```python
from build123d import *

# Parameters (mm, degrees)
F0_W     = 20
F0_H     = 20
F1_DEPTH = 20
F3_D     = 2
F5_D     = 2
F7_D     = 2


with BuildPart() as f1:
    # F0 (on Front) → F1 (new body)
    with BuildSketch(Plane.XZ):
        with Locations((10, 10)):
            Rectangle(F0_W, F0_H)
    extrude(amount=F1_DEPTH)

    # F3 (through all)
    with Locations(Plane.XZ.offset(20)):
        with Locations((10, 10)):
            Hole(F3_D / 2)

    # F5 (through all)
    with Locations(Plane.XY.offset(20)):
        with Locations((4.899733, -4.899733), (10, -10), (15.100267, -15.100267)):
            Hole(F5_D / 2)

    # F7 (through all)
    with Locations(Plane.YZ.offset(20)):
        with Locations((-10, 10), (-15.680383, 15.680383), (-15.680383, 4.319617), (-4.319617, 4.319617), (-4.319617, 15.680383)):
            Hole(F7_D / 2)


solid = f1.part
```
Geometry check sheet. Reference: the model listing, model coordinates, mm. Round coordinates to 2 decimals unless told otherwise and drop trailing zeros. Loops run counter-clockwise (first coordinate to the right, second up) from the corner with the lowest first, then second, coordinate; pieces in that order, holes last. Notation, with made-up numbers: M -29.5,-22.75 L 11.5,-22.75 A5 cw 11.5,-13.75 Z; hole C 56,-0.75 d1. An arc over 180 degrees is marked long. Return JSON: item names as keys, results as strings. Group by question number.
(1) Section check A-A, the plane y = -10. Enter the section's corners in (x, z).
(2) Section check C-C, the plane z = 15.25. Enter the section's corners in (x, y), and give its area (3 significant figures).
(3) Section check B-B, the plane x = 14.5. Enter the section's corners in (y, z), and give its area (3 significant figures).
(4) Scan lines: line 1 along Y through (x, z) = (3, 4.25); line 2 along Z through (x, y) = (10, -6); line 3 along Y through (x, z) = (3.5, 10). Record each from-to range of solid material in increasing order. Write a range as [from, to].
(5) Section check D-D, the plane y = -4.5. Enter the section's corners in (x, z), and give its area (3 significant figures).
(6) Mould release check, pull along X, two halves, no side actions. Record for faces 1 (the face through (9.86, -16.634, 4.62)), 2 (the face through (10, -15, 11)), 3 (the face through (20, -10, 12)): pulls with the +X half, pulls with the -X half, needs draft (parallel to the pull), parting line crosses it, or undercut.
(7) Go/stop test with flat-tipped pins: pin 1 (2.5 mm diameter, centred on x = 10, z = 10, fed in from +Y); pin 2 (1.2 mm diameter, centred on y = -10, z = 10, fed in from -X). Record where each tip stops, or that it passes through.
Data:
{
 "1": {"outline": "M 0,0 L 9,0 L 9,9 L 0,9 Z; M 0,11 L 9,11 L 9,20 L 0,20 Z; M 11,0 L 20,0 L 20,9 L 11,9 Z; M 11,11 L 20,11 L 20,20 L 11,20 Z"},
 "2": {"outline": "M 0,-20 L 20,-20 L 20,-16.58 L 0,-16.58 Z; M 0,-14.78 L 14.15,-14.78 A1 cw 16.05,-14.78 L 20,-14.78 L 20,-5.22 L 5.85,-5.22 A1 cw 3.95,-5.22 L 0,-5.22 Z; M 0,-3.42 L 20,-3.42 L 20,0 L 0,0 Z; hole C 10,-10 d2", "area": "323 mm²"},
 "3": {"outline": "M -20,0 L -15.9,0 L -15.9,3.34 A1 cw -15.9,5.3 L -15.9,14.7 A1 cw -15.9,16.66 L -15.9,20 L -20,20 Z; M -14.3,0 L 0,0 L 0,20 L -14.3,20 Z; hole C -10,10 d2; hole C -4.32,4.32 d2; hole C -4.32,15.68 d2", "area": "356 mm²"},
 "4": {"line 1": "[-20, -16.68], [-14.68, -5.32], [-3.32, 0]", "line 2": "[0, 9], [11, 20]", "line 3": "[-20, -11], [-9, 0]"},
 "5": {"outline": "M 0,0 L 3.98,0 L 3.98,3.34 L 0,3.34 Z; M 0,5.3 L 3.98,5.3 L 3.98,14.7 L 0,14.7 Z; M 0,16.66 L 3.98,16.66 L 3.98,20 L 0,20 Z; M 5.82,0 L 20,0 L 20,3.34 L 5.82,3.34 Z; M 5.82,5.3 L 20,5.3 L 20,14.7 L 5.82,14.7 Z; M 5.82,16.66 L 20,16.66 L 20,20 L 5.82,20 Z; hole C 10,10 d2", "area": "289 mm²"},
 "6": {"face 1": "needs draft", "face 2": "undercut", "face 3": "pulls with the +X half"},
 "7": {"pin 1": "y = 0", "pin 2": "through"}
}
